Verification items for the finished model (mm, model axes). A direction names the side the tool comes from. Give positions to 0.01 mm unless a question says otherwise; leave off trailing zeros. Write each loop counter-clockwise with the first axis right and the second up, starting at its lowest first coordinate (ties: lowest second). Pieces come first, ordered by that corner, then holes. Notation, with made-up numbers: (0, -25) - (5, -25) arc R26 cw to (5, -7) - close; hole circle Ø11 at (-17.75, 31.25). An arc over 180 degrees is marked (long way). Put each result on its own line as item: value.
from build123d import *

# Parameters (mm, degrees)
F0_R     = 6
F1_DEPTH = 119
F2_R     = 5
F3_DEPTH = 6
F4_R     = 3.5
F5_DEPTH = 10.13


with BuildPart() as f1:
    # F0 (on Right) → F1 (new body)
    with BuildSketch(Plane.YZ):
        Circle(F0_R)
    extrude(amount=F1_DEPTH)

    # F2 (on face) → F3 (join)
    with BuildSketch(Plane(origin=(0, 0, 0), x_dir=(0, -1, 0), z_dir=(-1, 0, 0))):
        Circle(F2_R)
    extrude(amount=F3_DEPTH)

    # F4 (on face) → F5 (join)
    with BuildSketch(Plane.YZ.offset(119)):
        Circle(F4_R)
    extrude(amount=F5_DEPTH)

    # F6 (on Front) → F7 (revolve)
    with BuildSketch(Plane.XZ):
        with BuildLine():
            Line((128, 0), (140, 0))
            ThreePointArc((140, 0), (134, 6), (128, 0))
        make_face()
    revolve(axis=Axis((134, 0, 0), (1, 0, 0)))


solid = f1.part
Q1. Set-up check for faces 1 (the face through (119, 3, -3)), 2 (the face through (0, -4, 4)), 3 (the face through (59, -6, 0)): record each of +Z, -Z, +X, -X, +Y, -Y from which the full face is reachable in a straight line by a thin tool's end or side.
Answers follow:
face 1: none
face 2: -X
face 3: +X, -X
Q2. Go/stop test with flat-tipped pins: pin 1 Ø6 at (x, y) = (48, 4) entering from -Z; pin 2 Ø6 at (x, z) = (100.5, -4.5) entering from +Y; pin 3 Ø1 at (x, z) = (70.5, 4) entering from -Y. Record where each tip stops, or that it passes through.
Answers follow:
pin 1: stops at z = -5.92
pin 2: stops at y = 5.81
pin 3: stops at y = -4.87
Q3. Scan lines: line 1 along X through (y, z) = (-2.25, -3.75); line 2 along Z through (x, y) = (96, 0.25); line 3 along X through (y, z) = (4, 3.5). Record each from-to range of solid material in increasing order.
Answers follow:
line 1: x = -6 to 119, 129.89 to 138.11
line 2: z = -5.99 to 5.99
line 3: x = 0 to 119, 131.22 to 136.78
Q4. Section check C-C, the plane x = 101.5. Record the cut outline in (y, z).
Answers follow:
outline: circle Ø12 at (0, 0)
Q5. Section check D-D, the plane x = 130.5. Record the cut outline in (y, z).
Answers follow:
outline: circle Ø9.75 at (0, 0)
Q6. Section check A-A, the plane y = 0. Record the cut outline in (x, z).
Answers follow:
outline: (-6, -5) - (0, -5) - (0, -6) - (119, -6) - (119, -3.5) - (129.13, -3.5) arc R6 ccw (long way) to (129.13, 3.5) - (119, 3.5) - (119, 6) - (0, 6) - (0, 5) - (-6, 5) - close
